Here's the drawing with two shaded views (mm, measured from the low corner). I have some questions. Round coordinates to 2 decimals unless told otherwise and drop trailing zeros. Loops run counter-clockwise (first coordinate to the right, second up) from the corner with the lowest first, then second, coordinate; pieces in that order, holes last. Notation, with made-up numbers: (84, 80) -> (124, 80) arc R22 cw to (124, 116) -> close; hole circle Ø8 at (33.5, 57.5). An arc over 180 degrees is marked (long way). Write each question's results on one line, items separated by ' | '. Start each with the question number.
1) Imagine slicing it at C-C, the plane x = 50.8. List the corners of the cut face in (y, z) for me (1 decimal).
2) Imagine slicing it at A-A, the plane x = 82.55. List the corners of the cut face in (y, z) for me (1 decimal), plus the area to 3 significant figures.
3) If I drill on probe 1 along Y at (x, z) = (50.8, 1.8) (1 decimal); probe 2 along X at (y, z) = (80, 1.55); probe 3 along Y at (x, z) = (19.05, 1.9) (1 decimal), over which ranges is the centre line in solid material (lowest first)?
4) Imagine slicing it at B-B, the plane y = 75. List the corners of the cut face in (x, z) for me (1 decimal).
5) Imagine slicing it at D-D, the plane z = 1.3. Give the number of separate pieces and of enclosed holes in the cut face, plus the area to 3 significant figures.
6) For P1, Ø2, axis at x = 80, y = 54.5, coming from the -Z side, with a flat end and sliding along its axis, tell me the tip position at first contact or that it passes through.
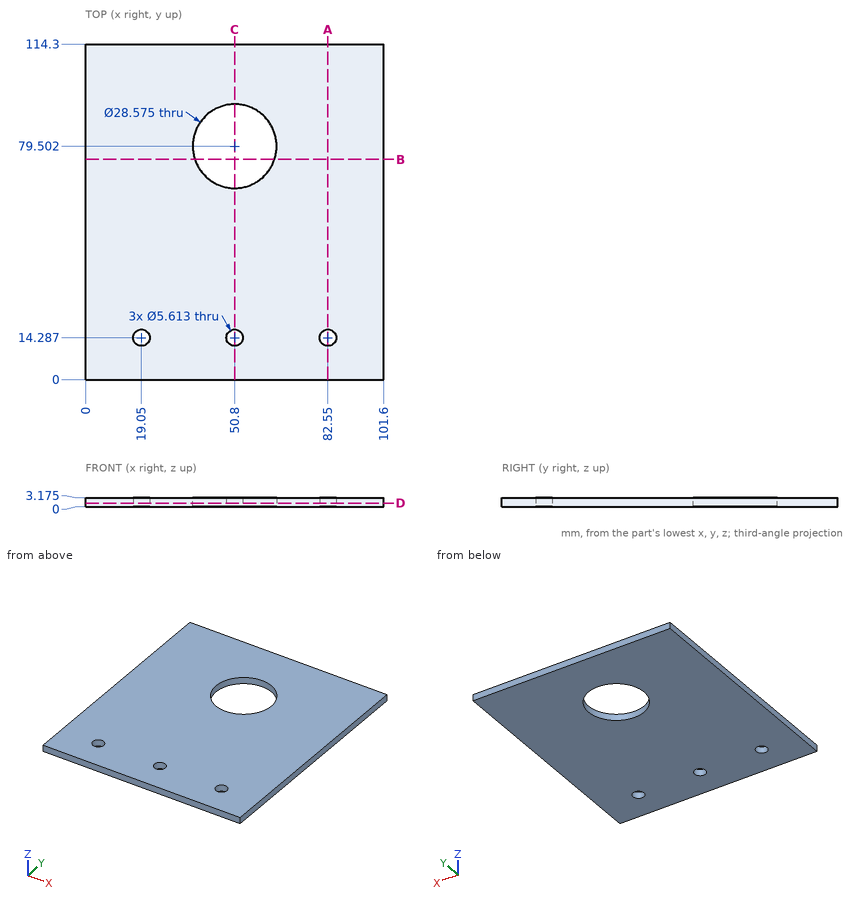
Checked values:
1) outline: (0, 0) -> (11.5, 0) -> (11.5, 3.2) -> (0, 3.2) -> close; (17.1, 0) -> (65.2, 0) -> (65.2, 3.2) -> (17.1, 3.2) -> close; (93.8, 0) -> (114.3, 0) -> (114.3, 3.2) -> (93.8, 3.2) -> close
2) outline: (0, 0) -> (11.5, 0) -> (11.5, 3.2) -> (0, 3.2) -> close; (17.1, 0) -> (114.3, 0) -> (114.3, 3.2) -> (17.1, 3.2) -> close | area: 345 mm^2
3) probe 1: 0 to 11.5, 17.1 to 65.2, 93.8 to 114.3 | probe 2: 0 to 36.52, 65.08 to 101.6 | probe 3: 0 to 11.5, 17.1 to 114.3
4) outline: (0, 0) -> (37.2, 0) -> (37.2, 3.2) -> (0, 3.2) -> close; (64.4, 0) -> (101.6, 0) -> (101.6, 3.2) -> (64.4, 3.2) -> close
5) separate pieces: 1 | enclosed holes: 4 | area: 10,900 mm^2
6) P1: z = 0
